For this review, take the finished solid that the model builds, in its own axes (mm). Face numbers are marked on the shaded views. A direction names the side the tool comes from. Round coordinates to 2 decimals unless told otherwise and drop trailing zeros. Loops run counter-clockwise (first coordinate to the right, second up) from the corner with the lowest first, then second, coordinate; pieces in that order, holes last.
1. Tool access review of the marked faces 5, 6 and 7: name each direction out of +Z, -Z, +X, -X, +Y, -Y from which nothing blocks a thin tool from reaching the whole face with its end or side.
2. Consider section A-A on x = 63. State the section outline as (y, z) points, then the cut area to 3 significant figures.
3. Draft analysis for pull direction Y (two halves, no side actions). For the marked faces 1, 2, 3 and 4, state which applies: released by +Y, released by -Y, zero draft, split by the parting line, or undercut.
4. Consider section C-C on y = 13. State the section outline as (x, z) points.
5. Consider section B-B on z = 10.25. State the section outline as (x, y) points.
6. To check wall thickness, follow line 1 along Y through (x, z) = (25, 2.25); line 2 along Y through (x, z) = (10, 11); line 3 along X through (y, z) = (36.5, 13.5). State the ranges of each line that lie inside material, in increasing order.
7. Consider section D-D on x = 32.5. State the section outline as (y, z) points.
8. Clearance check with flat-ended pins moving along their axes: pin 1 Ø1.5 at (y, z) = (107.5, 10) entering from -X; pin 2 Ø8 at (x, z) = (28.5, 6) entering from +Y; pin 3 Ø1.1 at (y, z) = (114.5, 13.5) entering from -X. State where each tip first meets the part, or that it passes through.
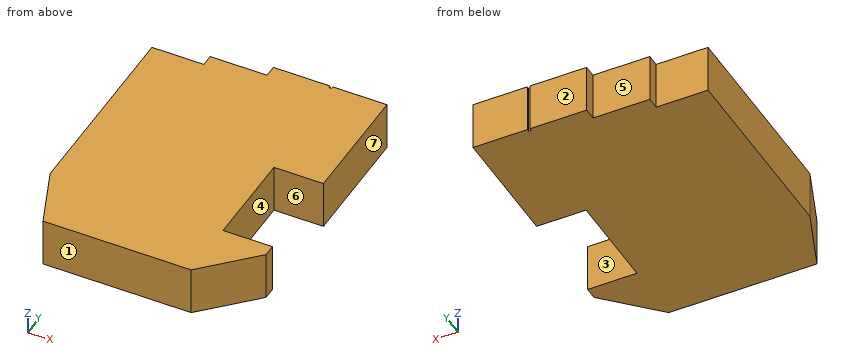
from build123d import *

# Parameters (mm, degrees)
BOSS_EXTRUDE1_DEPTH = 20
SKETCH2_W           = 20
SKETCH2_H           = 40
CUT_EXTRUDE1_DEPTH  = 142.509716981


with BuildPart() as part:
    # Sketch1 → Boss-Extrude1 (new body)
    with BuildSketch(Plane.XY):
        Polygon((58, 114), (58, 115), (80, 115), (80, 20), (60, 0), (0, 0), (-10, 25), (-10, 105), (11, 105), (11, 110), (12, 110), (34, 110), (34, 115), (35, 115), (57, 115), (57, 114), align=None)
    extrude(amount=BOSS_EXTRUDE1_DEPTH)

    # Sketch2 → Cut-Extrude1 (cut, through all)
    with BuildSketch(Plane.XY.offset(20)):
        with Locations((70, 45)):
            Rectangle(SKETCH2_W, SKETCH2_H)
    extrude(amount=-CUT_EXTRUDE1_DEPTH, mode=Mode.SUBTRACT)


solid = part.part
Resolved:
1. face 5: +Z, -Z, -X, +Y
1. face 6: +Z, -Z, +X
1. face 7: +Z, -Z, +X, +Y, -Y
2. outline: (3, 0) - (25, 0) - (25, 20) - (3, 20) - close; (65, 0) - (115, 0) - (115, 20) - (65, 20) - close
2. area: 1,440 mm2
3. face 1: released by -Y
3. face 2: released by +Y
3. face 3: undercut
3. face 4: undercut
4. outline: (-5.2, 0) - (73, 0) - (73, 20) - (-5.2, 20) - close
5. outline: (-10, 25) - (0, 0) - (60, 0) - (80, 20) - (80, 25) - (60, 25) - (60, 65) - (80, 65) - (80, 115) - (58, 115) - (58, 114) - (57, 114) - (57, 115) - (34, 115) - (34, 110) - (11, 110) - (11, 105) - (-10, 105) - close
6. line 1: y = 0 to 110
6. line 2: y = 0 to 105
6. line 3: x = -10 to 60
7. outline: (0, 0) - (110, 0) - (110, 20) - (0, 20) - close
8. pin 1: stops at x = 11
8. pin 2: stops at y = 110
8. pin 3: stops at x = 34
